The listing builds one solid part. Answer for the finished solid, in the listing's coordinates (mm). A direction names the side the tool comes from. Coordinates: 2 decimals unless noted, no trailing zeros. Write each loop counter-clockwise with the first axis right and the second up, starting at its lowest first coordinate (ties: lowest second). Pieces come first, ordered by that corner, then holes. Notation, with made-up numbers: M 45,58 L 72,58 A23 cw 72,91 Z; hole C 13.25,48.5 d6. An arc over 180 degrees is marked long. Answer as CSV lines item,"result". Start each with the question number.
```python
from build123d import *

# Parameters (mm, degrees)
F1_DEPTH = 38.1
F2_R     = 3.175
F3_DEPTH = 177.8
F4_R     = 6.35
F6_DEPTH = 12.7
F7_R     = 12.7


with BuildPart() as f1:
    # F0 (on Front) → F1 (new body)
    with BuildSketch(Plane.XZ):
        Polygon((-44.45, 13.515173), (-44.45, 8.739973), (-25.4, 8.530632), (-25.4, -0.994368), (-44.45, -0.994368), (-44.45, -5.534827), (0, -5.534827), (0, 13.515173), align=None)
    extrude(amount=-F1_DEPTH)

    # F2 (on face) → F3 (cut)
    with BuildSketch(Plane.XY.offset(13.515173)):
        with Locations((-34.925, 28.575)):
            Circle(F2_R)
        with Locations((-34.925, 9.525)):
            Circle(F2_R)
    extrude(amount=-F3_DEPTH, mode=Mode.SUBTRACT)

    # F4
    f4_edges = [f1.edges().sort_by_distance(p)[0] for p in [
        (-44.45, 38.1, 11.127573),
        (-44.45, 38.1, -3.264598),
        (-44.45, 0, 11.127573),
        (-44.45, 0, -3.264598),
    ]]
    fillet(f4_edges, radius=F4_R)

    # F5 (on face) → F6 (cut)
    with BuildSketch(Plane.YZ):
        with BuildLine():
            ThreePointArc((25.4, 3.990173), (19.05, 10.340173), (12.7, 3.990173))
            Line((12.7, 3.990173), (25.4, 3.990173))
        make_face()
        with BuildLine():
            Line((25.4, 3.990173), (12.7, 3.990173))
            ThreePointArc((12.7, 3.990173), (19.05, -2.359827), (25.4, 3.990173))
        make_face()
    extrude(amount=-F6_DEPTH, mode=Mode.SUBTRACT)

    # F7
    f7_edges = [f1.edges().sort_by_distance(p)[0] for p in [
        (-25.4, 0, 3.768132),
        (-25.4, 38.1, 3.768132),
    ]]
    fillet(f7_edges, radius=F7_R)


solid = f1.part
```
1) The part is cut by section B-B (z = 11.5). Determine the outline of the cut face in (x, y) (3 decimals).
2) Which of the six approach directions +Z, -Z, +X, -X, +Y, -Y give full straight-line access (tool end or side, diameter ignored) to faces 1 (the face through (-25.4, 19, 4)), 2 (the face through (-21.58, 3.62, 3.7)), 3 (the face through (-11, 38.1, 4))?
3) Find the intervals of material crossed by line 1 (Z direction, x = -26, y = 26.5); line 2 (X direction, y = 28.5, z = 9.75); line 3 (Y direction, x = -9.5, z = 4), in increasing order. Write a range as from..to.
4) Each of these flat-tipped pins is pushed along its axis until it touches: P1, Ø5.5, axis at x = -34.925, y = 28.575, coming from the +Z side; P2, Ø7.5, axis at y = 21, z = 4, coming from the -X side; P3, Ø6.5, axis at y = 20.5, z = 3, coming from the +X side. Where does it stop, or does it pass through?
5) The part is cut by section A-A (y = 27). Determine the outline of the cut face in (x, z) (3 decimals), then the cut area to 3 significant figures.
6) The part is cut by section D-D (y = 19.05). Determine the outline of the cut face in (x, z), then the cut area to 3 significant figures.
7) For a pull along X with two mould halves and no side action, classify faces 4 (the face through (-21.58, 34.48, 3.7)), 5 (the face through (-33.46, 25.76, -3.23)), 6 (the face through (-33.218, 12.202, 11.092)), 7 (the face through (-22, 19, 13.515)) as +X half, -X half, draft (parallel to the pull), parting line (faces both ways), or undercut.
8) The part is cut by section C-C (x = -27). Determine the outline of the cut face in (y, z).
Completed:
1,outline,"M -44.45,6.35 A6.35 ccw -38.1,0 L 0,0 L 0,38.1 L -38.1,38.1 A6.35 ccw -44.45,31.75 Z; hole C -34.925,9.525 d6.35; hole C -34.925,28.575 d6.35"
2,face 1,"-X, +Y, -Y"
2,face 2,"-X, -Y"
2,face 3,"+Z, -Z, +X, -X, +Y"
3,line 1,"-5.53..-0.99, 8.54..13.52"
3,line 2,"-44.45..-38.1, -31.75..0"
3,line 3,"0..12.7, 25.4..38.1"
4,P1,"through"
4,P2,"x = -25.4"
4,P3,"x = -12.7"
5,outline,"M -44.45,-5.535 L -37.682,-5.535 L -37.682,-0.994 L -44.45,-0.994 Z; M -44.45,8.74 L -37.682,8.666 L -37.682,13.515 L -44.45,13.515 Z; M -32.168,-5.535 L 0,-5.535 L 0,13.515 L -32.168,13.515 L -32.168,8.605 L -25.299,8.53 L -25.299,-0.994 L -32.168,-0.994 Z"
5,area,"610 mm²"
6,outline,"M -44.45,-5.53 L 0,-5.53 L 0,-2.36 L -12.7,-2.36 L -12.7,10.34 L 0,10.34 L 0,13.52 L -44.45,13.52 L -44.45,8.74 L -25.4,8.53 L -25.4,-0.99 L -44.45,-0.99 Z"
6,area,"502 mm²"
7,face 4,"-X half"
7,face 5,"undercut"
7,face 6,"undercut"
7,face 7,"draft"
8,outline,"M 0,-5.53 L 38.1,-5.53 L 38.1,-0.99 L 0,-0.99 Z; M 0,8.55 L 38.1,8.55 L 38.1,13.52 L 0,13.52 Z"
